from build123d import *

# Parameters (mm, degrees)
SKETCH1_W             = 50.8
SKETCH1_H             = 25.4
SKETCH1_W_2           = 45.72
SKETCH1_H_2           = 20.32
BOSS_EXTRUDE1_DEPTH   = 533.4
F_8_CLEARANCE_HOLE1_D = 4.4958
CUT_EXTRUDE2_DEPTH    = 76.962


with BuildPart() as part:
    # Sketch1 → Boss-Extrude1 (new body)
    with BuildSketch(Plane.XY):
        Rectangle(SKETCH1_W, SKETCH1_H)
        Rectangle(SKETCH1_W_2, SKETCH1_H_2, mode=Mode.SUBTRACT)
    extrude(amount=-BOSS_EXTRUDE1_DEPTH)

    # #8 Clearance Hole1 (through all)
    with Locations(Plane(origin=(25.4, 0, 0), x_dir=(0, 0, -1), z_dir=(1, 0, 0))):
        with Locations((12.7, 0), (38.1, 0), (63.5, 0), (88.9, 0), (114.3, 0), (139.7, 0), (165.1, 0), (190.5, 0), (215.9, 0), (241.3, 0), (266.7, 0), (292.1, 0), (317.5, 0), (342.9, 0), (368.3, 0), (393.7, 0), (419.1, 0), (444.5, 0), (469.9, 0), (495.3, 0), (520.7, 0)):
            Hole(F_8_CLEARANCE_HOLE1_D / 2)

    # Sketch4 → Cut-Extrude2 (cut)
    with BuildSketch(Plane(origin=(0, 12.7, 0), x_dir=(1, 0, 0), z_dir=(0, 1, 0))):
        Polygon((-7.206301081, 228.6), (135.513081356, 228.6), (135.513081356, -17.641370014), (-94.056886123, -17.641370014), (-94.056886123, 228.6), align=None)
    extrude(amount=-CUT_EXTRUDE2_DEPTH, mode=Mode.SUBTRACT)


solid = part.part
Check sheet for the modelled part. Datum: model origin and axes. Units: mm. A direction names the side the tool comes from. Coordinates: 2 decimals unless noted, no trailing zeros. Write each loop counter-clockwise with the first axis right and the second up, starting at its lowest first coordinate (ties: lowest second). Pieces come first, ordered by that corner, then holes.
Item 1: Access from +Z, -Z, +X, -X, +Y, -Y to the whole of each face (thin tool, end or side, straight path). Record for faces 1 (the face through (0, -10.16, -379)), 2 (the face through (0, 12.7, -379)).
Numbers:
face 1: +Z, -Z
face 2: +Z, -Z, +X, -X, +Y
Item 2: Depth check by flat-ended pin: pin 1 Ø3.5 at (y, z) = (0, -266.7) entering from -X. Enter the tip coordinate at first touch or a pass-through.
Numbers:
pin 1: passes through
Item 3: Cross-section at B-B on y = -5.75. Record the boundary of the cut face in (x, z).
Numbers:
outline: (-25.4, -533.4) - (-22.86, -533.4) - (-22.86, -228.6) - (-25.4, -228.6) - close; (22.86, -533.4) - (25.4, -533.4) - (25.4, -228.6) - (22.86, -228.6) - close
Item 4: Scan lines: probe 1 along X at (y, z) = (1, -277.5); probe 2 along Y at (x, z) = (-23, -368); probe 3 along Y at (x, z) = (2, -475.5). Record each from-to range of solid material in increasing order.
Numbers:
probe 1: x = -25.4 to -22.86, 22.86 to 25.4
probe 2: y = -12.7 to -2.23, 2.23 to 12.7
probe 3: y = -12.7 to -10.16, 10.16 to 12.7
Item 5: Cross-section at C-C on z = -285. Record the boundary of the cut face in (x, y), then the cut area to 3 significant figures.
Numbers:
outline: (-25.4, -12.7) - (25.4, -12.7) - (25.4, 12.7) - (-25.4, 12.7) - close; hole (-22.86, -10.16) - (22.86, -10.16) - (22.86, 10.16) - (-22.86, 10.16) - close
area: 361 mm2
Item 6: Mould release check, pull along X, two halves, no side actions. Record for faces 3 (the face through (25.4, 0, -379)), 4 (the face through (0, -12.7, -379)), 5 (the face through (22.86, 0, -379)), 6 (the face through (0, 10.16, -379)): released by +X, released by -X, zero draft, split by the parting line, or undercut.
Numbers:
face 3: released by +X
face 4: zero draft
face 5: undercut
face 6: undercut
Item 7: Cross-section at A-A on x = 6. Record the boundary of the cut face in (y, z), then the cut area to 3 significant figures.
Numbers:
outline: (-12.7, -533.4) - (-10.16, -533.4) - (-10.16, -228.6) - (-12.7, -228.6) - close; (10.16, -533.4) - (12.7, -533.4) - (12.7, -228.6) - (10.16, -228.6) - close
area: 1,550 mm2
